from build123d import *

# Parameters (mm, degrees)
SKETCH_1_R               = 326
EXTRUDE_1_DEPTH          = 1.5
SKETCH_3_R               = 10
EXTRUDE_2_DEPTH          = 6
CUT_EXTRUDE_1_DEPTH      = 462.072662386
CUT_EXTRUDE_1_DEPTH_BACK = 462.072662386
SKETCH_4_R               = 53


with BuildPart() as part:
    # 草图1 → 凸台-拉伸1 (new, symmetric)
    with BuildSketch(Plane(origin=(0, 0, 0), x_dir=(1, 0, 0), z_dir=(0, 1, 0))):
        with Locations(Location((0, 0, 0), (0, 0, 270))):
            Circle(SKETCH_1_R)
    extrude(amount=EXTRUDE_1_DEPTH, both=True)

    # 草图3 → 凸台-拉伸2 (add)
    with BuildSketch(Plane(origin=(0, 0, 0), x_dir=(1, 0, 0), z_dir=(0, 1, 0))):
        with Locations(Location((0, 0, 0), (0, 0, 270))):
            Circle(SKETCH_3_R)
    extrude(amount=-EXTRUDE_2_DEPTH)

    # 草图4 → 切除-拉伸1 (cut, two sides: drawn at the far end of the back side and taken through both)
    with BuildSketch(Plane(origin=(0, 0, 0), x_dir=(1, 0, 0), z_dir=(0, 1, 0)).offset(-CUT_EXTRUDE_1_DEPTH_BACK)):
        with Locations(Location((233, 0, 0), (0, 0, 270))):
            Circle(SKETCH_4_R)
    extrude(amount=CUT_EXTRUDE_1_DEPTH + CUT_EXTRUDE_1_DEPTH_BACK, mode=Mode.SUBTRACT)


solid = part.part
The model under review builds one solid part; all positions refer to its coordinate system, in mm. A direction names the side the tool comes from. Give positions to 0.01 mm unless a question says otherwise; leave off trailing zeros. Loops run counter-clockwise (first coordinate to the right, second up) from the corner with the lowest first, then second, coordinate; pieces in that order, holes last. Notation, with made-up numbers: (8.25, 11) -> (33.25, 11) arc R9 cw to (33.25, 27) -> close; hole circle Ø9 at (82.25, -13). An arc over 180 degrees is marked (long way). Write each question's results on one line, items separated by ' | '.
1) For line 1 along X through (y, z) = (0.8, 0); line 2 along Y through (x, z) = (-39, -229.5); line 3 along Z through (x, y) = (235.5, -0.25), list the stretches that pass through material, from the lowest coordinate up. Write a range as from..to.
Conclusion:
line 1: x = -326..180, 286..326 | line 2: y = -1.5..1.5 | line 3: z = -225.42..-52.94, 52.94..225.42
2) Insertion check: pin 1 Ø2 at (x, z) = (202, -241.5) entering from -Y; pin 2 Ø1 at (x, y) = (-84, -1.5) entering from -Z (3 decimals). Each pin has a flat end and moves straight along its axis. Give the tip position at first contact, or say it passes through.
Conclusion:
pin 1: stops at y = -1.5 | pin 2: stops at z = -315.125
3) Draft analysis for pull direction Z (two halves, no side actions). For faces 1 (the face through (5, 1.5, -5)), 2 (the face through (-124.86, 0.02, 301.14)), 3 (the face through (181.26, -0.02, -11.49)), state which applies: pulls with the +Z half, pulls with the -Z half, needs draft (parallel to the pull), parting line crosses it, or undercut.
Conclusion:
face 1: needs draft | face 2: parting line crosses it | face 3: undercut
4) Take a section at B-B, the plane x = 0. Give the boundary of the cut face in (y, z), plus the area to 3 significant figures.
Conclusion:
outline: (-6, -10) -> (-1.5, -10) -> (-1.5, -326) -> (1.5, -326) -> (1.5, 326) -> (-1.5, 326) -> (-1.5, 10) -> (-6, 10) -> close | area: 2,050 mm^2
5) Take a section at D-D, the plane y = -4.5. Give the boundary of the cut face in (x, z).
Conclusion:
outline: circle Ø20 at (0, 0)
6) Take a section at C-C, the plane x = 233. Give the boundary of the cut face in (y, z), plus the area to 3 significant figures.
Conclusion:
outline: (-1.5, -228.01) -> (1.5, -228.01) -> (1.5, -53) -> (-1.5, -53) -> close; (-1.5, 53) -> (1.5, 53) -> (1.5, 228.01) -> (-1.5, 228.01) -> close | area: 1,050 mm^2
7) Take a section at A-A, the plane z = 0. Give the boundary of the cut face in (x, y), plus the area to 3 significant figures.
Conclusion:
outline: (-326, -1.5) -> (-10, -1.5) -> (-10, -6) -> (10, -6) -> (10, -1.5) -> (180, -1.5) -> (180, 1.5) -> (-326, 1.5) -> close; (286, -1.5) -> (326, -1.5) -> (326, 1.5) -> (286, 1.5) -> close | area: 1,730 mm^2
8) Tool access review of faces 4 (the face through (0, -6, 0)), 5 (the face through (-9.76, -3.72, -2.17)): name each direction out of +Z, -Z, +X, -X, +Y, -Y from which nothing blocks a thin tool from reaching the whole face with its end or side.
Conclusion:
face 4: +Z, -Z, +X, -X, -Y | face 5: -Y
